Build history of the part. All positions in model axes, mm. Round coordinates to 2 decimals unless told otherwise and drop trailing zeros. Order: outer loops, then holes, each group sorted by start corner. A loop starts at its lowest first (then second) coordinate and runs counter-clockwise, first axis right, second up. Notation, with made-up numbers: (65, 28.25) -> (92, 28.25) arc R9 ccw to (92, 45.25) -> close; hole circle Ø4 at (78.5, 53.25). An arc over 180 degrees is marked (long way). Answer as CSV lines item,"result". Start each with the question number.
```python
from build123d import *

# Parameters (mm, degrees)
BOSS_EXTRUDE1_DEPTH = 3
SKETCH3_R           = 3
CUT_EXTRUDE1_DEPTH  = 10
SKETCH4_R           = 4.62
CUT_EXTRUDE2_DEPTH  = 10
SKETCH5_W           = 140
SKETCH5_H           = 1
CUT_EXTRUDE3_DEPTH  = 80


with BuildPart() as part:
    # Sketch1 → Boss-Extrude1 (new body)
    with BuildSketch(Plane(origin=(0, 0, 0), x_dir=(1, 0, 0), z_dir=(0, 1, 0))):
        with BuildLine():
            Line((70, 28.5), (70, -32.5))
            Line((70, -32.5), (-70, -32.5))
            Line((-70, -32.5), (-70, 28.5))
            ThreePointArc((-70, 28.5), (0, 38.554020598), (70, 28.5))
        make_face()
    extrude(amount=BOSS_EXTRUDE1_DEPTH)

    # Sketch3 → Cut-Extrude1 (cut)
    with BuildSketch(Plane(origin=(0, 3, 0), x_dir=(1, 0, 0), z_dir=(0, 1, 0))):
        with Locations(Location((-63, 25, 0), (0, 0, 270))):
            Circle(SKETCH3_R)
        with Locations(Location((-63, -27, 0), (0, 0, 270))):
            Circle(SKETCH3_R)
        with Locations(Location((63, 25, 0), (0, 0, 270))):
            Circle(SKETCH3_R)
        with Locations(Location((63, -27, 0), (0, 0, 270))):
            Circle(SKETCH3_R)
    extrude(amount=-CUT_EXTRUDE1_DEPTH, mode=Mode.SUBTRACT)

    # Sketch4 → Cut-Extrude2 (cut)
    with BuildSketch(Plane(origin=(0, 3, 0), x_dir=(1, 0, 0), z_dir=(0, 1, 0))):
        with Locations(Location((-23.33, -4.5, 0), (0, 0, 270))):
            Circle(SKETCH4_R)
        with Locations(Location((22.67, -4.5, 0), (0, 0, 270))):
            Circle(SKETCH4_R)
        with Locations(Location((-0.33, 20.499217988, 0), (0, 0, 270))):
            Circle(SKETCH4_R)
    extrude(amount=-CUT_EXTRUDE2_DEPTH, mode=Mode.SUBTRACT)

    # Sketch5 → Cut-Extrude3 (cut)
    with BuildSketch(Plane.XY.offset(32.5)):
        with Locations((0, 0.5)):
            Rectangle(SKETCH5_W, SKETCH5_H)
    extrude(amount=-CUT_EXTRUDE3_DEPTH, mode=Mode.SUBTRACT)


solid = part.part
```
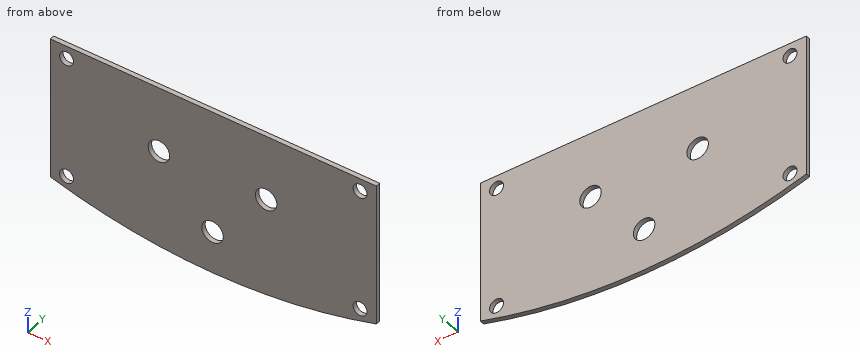
Q1. Slice it at D-D, the plane x = 63. Write the cut outline in (y, z), plus the area to 3 significant figures.
Q2. Slice it at A-A, the plane x = -0.33. Write the cut outline in (y, z), plus the area to 3 significant figures.
Q3. Probe L1, parallel to X at y = 2.2, z = 4.5; L2, parallel to X at y = 1.9, z = 8; L3, parallel to Z at x = 26, y = 2.05. List the from-to ranges inside material, lowest first.
Q4. Flat gauge pin, fed straight in: pin 1 Ø9.5 at (x, z) = (63, -25) entering from +Y. Where does the tip first touch, or does it go through?
Q5. Slice it at C-C, the plane y = 1.45. Write the cut outline in (x, z).
Q6. Slice it at B-B, the plane z = 1.5. Write the cut outline in (x, y), plus the area to 3 significant figures.
Solutions:
1,outline,"(1, -30.44) -> (3, -30.44) -> (3, -28) -> (1, -28) -> close; (1, -22) -> (3, -22) -> (3, 24) -> (1, 24) -> close; (1, 30) -> (3, 30) -> (3, 32.5) -> (1, 32.5) -> close"
1,area,"102 mm2"
2,outline,"(1, -38.55) -> (3, -38.55) -> (3, -25.12) -> (1, -25.12) -> close; (1, -15.88) -> (3, -15.88) -> (3, 32.5) -> (1, 32.5) -> close"
2,area,"124 mm2"
3,L1,"x = -70 to -27.95, -18.71 to 18.05, 27.29 to 70"
3,L2,"x = -70 to -26.35, -20.31 to 19.65, 25.69 to 70"
3,L3,"z = -37.19 to 1.3, 7.7 to 32.5"
4,pin 1,"stops at y = 3"
5,outline,"(-70, -28.5) arc R248.71 ccw to (70, -28.5) -> (70, 32.5) -> (-70, 32.5) -> close; hole circle Ø6 at (-63, -25); hole circle Ø6 at (-63, 27); hole circle Ø9.24 at (-23.33, 4.5); hole circle Ø9.24 at (-0.33, -20.5); hole circle Ø9.24 at (22.67, 4.5); hole circle Ø6 at (63, -25); hole circle Ø6 at (63, 27)"
6,outline,"(-70, 1) -> (-26.84, 1) -> (-26.84, 3) -> (-70, 3) -> close; (-19.82, 1) -> (19.16, 1) -> (19.16, 3) -> (-19.82, 3) -> close; (26.18, 1) -> (70, 1) -> (70, 3) -> (26.18, 3) -> close"
6,area,"252 mm2"
